The listing builds one solid part. Answer for the finished solid, in the listing's coordinates (mm). Face numbers are marked on the shaded views. A direction names the side the tool comes from. Round coordinates to 2 decimals unless told otherwise and drop trailing zeros. Write each loop counter-clockwise with the first axis right and the second up, starting at its lowest first coordinate (ties: lowest second). Pieces come first, ordered by that corner, then holes. Notation, with made-up numbers: M 2.25,-28 L 9.25,-28 A12 ccw 9.25,-19 Z; hole C 60.5,15.25 d5. An arc over 180 degrees is marked long. One line per item, written item: value. Start each with the question number.
(1) Given P1, Ø3, axis at x = 0, z = 0, coming from the +Y side; P2, Ø1, axis at y = 9, z = 3, coming from the +X side; P3, Ø5, axis at y = 5, z = -4.5, coming from the -X side; P4, Ø2.5, axis at x = 1.5, z = -1, coming from the -Y side, each flat-ended and moving along its own axis, determine where each tip first touches the part or whether it passes through.
(2) For the marked faces 1 and 2, determine the directions among +Z, -Z, +X, -X, +Y, -Y from which every point of the face is accessible in a straight line to the end or side of a thin tool.
(3) Section A-A (y = 13) is taken. Determine the outline of the cut face in (x, z).
(4) Consider probe 1 along X at (y, z) = (10.3, 0); probe 2 along X at (y, z) = (5.25, 0). Determine where each line is inside the solid, lowest interval first.
(5) For a pull along X with two mould halves and no side action, classify the marked faces 3, 4, 5 and 6 as released by +X, released by -X, zero draft, split by the parting line, or undercut.
(6) Section B-B (y = 5.25) is taken. Determine the outline of the cut face in (x, z).
```python
from build123d import *

# Parameters (mm, degrees)
SKETCH1_R           = 7.5
SKETCH1_R_2         = 4.5
BOSS_EXTRUDE1_DEPTH = 10
SKETCH2_R           = 7.5
SKETCH2_R_2         = 2.65
BOSS_EXTRUDE2_DEPTH = 6
CUT_EXTRUDE1_DEPTH  = 4.5
FILLET1_R           = 3
FILLET2_R           = 1


with BuildPart() as part:
    # Sketch1 → Boss-Extrude1 (new body)
    with BuildSketch(Plane(origin=(0, 0, 0), x_dir=(1, 0, 0), z_dir=(0, 1, 0))):
        with Locations(Location((0, 0, 0), (0, 0, 270))):
            Circle(SKETCH1_R)
        with Locations(Location((0, 0, 0), (0, 0, 270))):
            Circle(SKETCH1_R_2, mode=Mode.SUBTRACT)
    extrude(amount=BOSS_EXTRUDE1_DEPTH)

    # Sketch2 → Boss-Extrude2 (add)
    with BuildSketch(Plane(origin=(0, 10, 0), x_dir=(1, 0, 0), z_dir=(0, 1, 0))):
        with Locations(Location((0, 0, 0), (0, 0, 270))):
            Circle(SKETCH2_R)
        with Locations(Location((0, 0, 0), (0, 0, 270))):
            Circle(SKETCH2_R_2, mode=Mode.SUBTRACT)
    extrude(amount=BOSS_EXTRUDE2_DEPTH)

    # Sketch3 → Cut-Extrude1 (cut)
    with BuildSketch(Plane(origin=(0, 16, 0), x_dir=(1, 0, 0), z_dir=(0, 1, 0))):
        Polygon((2.598076211, 4.5), (-2.598076211, 4.5), (-5.196152423, 0), (-2.598076211, -4.5), (2.598076211, -4.5), (5.196152423, 0), align=None)
    extrude(amount=-CUT_EXTRUDE1_DEPTH, mode=Mode.SUBTRACT)

    # Fillet1
    fillet1_edges = [part.edges().sort_by_distance(p)[0] for p in [
        (0, 0, -7.5),
    ]]
    fillet(fillet1_edges, radius=FILLET1_R - 0.0001)  # a hair under: the kernel refuses the full size

    # Fillet2
    fillet2_edges = [part.edges().sort_by_distance(p)[0] for p in [
        (0, 0, -4.5),
    ]]
    fillet(fillet2_edges, radius=FILLET2_R)


solid = part.part
```
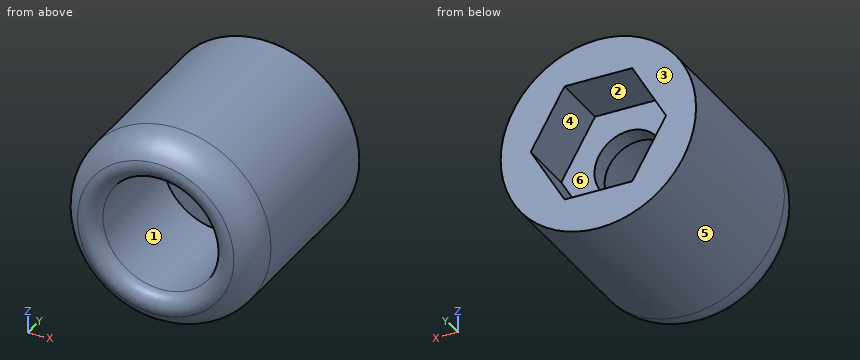
Recorded:
1. P1: passes through
1. P2: stops at x = 7.07
1. P3: stops at x = -7.23
1. P4: stops at y = 10
2. face 1: -Y
2. face 2: +Y
3. outline: C 0,0 d15; hole M -5.2,0 L -2.6,-4.5 L 2.6,-4.5 L 5.2,0 L 2.6,4.5 L -2.6,4.5 Z
4. probe 1: x = -7.5 to -2.65, 2.65 to 7.5
4. probe 2: x = -7.5 to -4.5, 4.5 to 7.5
5. face 3: zero draft
5. face 4: undercut
5. face 5: split by the parting line
5. face 6: undercut
6. outline: C 0,0 d15; hole C 0,0 d9
